Check sheet for the modelled part. Datum: model origin and axes. Units: mm. A direction names the side the tool comes from. Round coordinates to 2 decimals unless told otherwise and drop trailing zeros. Order: outer loops, then holes, each group sorted by start corner. A loop starts at its lowest first (then second) coordinate and runs counter-clockwise, first axis right, second up. Notation, with made-up numbers: (-15, -25.5) -> (32, -25.5) arc R16 cw to (32, -19.5) -> close; hole circle Ø8 at (24.25, 51). An arc over 180 degrees is marked (long way). Answer in a Markdown table with one row per item.
Autodesk Fusion 360 part; units mm, degrees
sketch "スケッチ1" plane through (0, 0, 0) normal (0, 0, 1) x (1, 0, 0)
  line L0 (0, 0) -> (72.6, 0)
  line L1 (72.6, 0) -> (72.6, -36.25)
  line L2 (72.6, -36.25) -> (0, -36.25)
  line L3 (0, -36.25) -> (0, 0)
  line L4 (36.3, 0) -> (36.3, -36.25)
  line L5 (0, -18.125) -> (72.6, -18.125)
  line L6 (72.6, -8.625) -> (72.6, -26.625)
  line L7 (58.3, -36.25) -> (14.3, -36.25)
  line L8 (0, -9.125) -> (0, -27.125)
  line L9 (0, -18.125) -> (9.5, -18.125)
  line L10 (0, -9.125) -> (6.4586, -9.125)
  line L11 (0, -27.125) -> (4.6488, -27.125)
  line L12 (6.4586, -9.125) -> (36.3, 0)
  line L13 (14.3, -36.25) -> (12.3, -36.25)
  line L14 (12.3, -36.25) -> (2.2204, -24.2289)
  line L15 (36.3, -18.125) -> (36.3, -32.425)
  line L16 (36.3, -18.125) -> (36.3, -3.825)
  line L17 (66.1414, -9.125) -> (36.3, 0)
  line L18 (60.3, -36.25) -> (70.3796, -24.2289)
  line L19 (58.3, -36.25) -> (60.3, -36.25)
  line L20 (6.4586, -27.125) -> (66.1414, -27.125)
  line L21 (6.4586, -9.125) -> (66.1414, -9.125)
  arc A0 (6.9878, -8.9632) -> (6.4586, -27.125) centre (9.5, -18.125) ccw
  arc A1 (66.1414, -27.125) -> (65.6122, -8.9632) centre (63.1, -18.125) ccw
  circle A2 centre (14.3, -32.425) radius 1.75
  circle A3 centre (36.3, -3.825) radius 1.75
  circle A4 centre (58.3, -32.425) radius 1.75
  circle A5 centre (32.3, -32.425) radius 1
  circle A6 centre (40.3, -32.425) radius 1
  point P0 (36.3, -18.125)
  point P1 (36.3, -3.825)
  point P2 (14.3, -32.425)
  point P3 (58.3, -32.425)
  point P4 (40.3, -32.425)
  point P5 (40.3, -32.425)
  point P6 (32.3, -32.425)
  dimension "d5" = 72.6
  dimension "d6" = 36.25
  dimension "d10" = 44
  dimension "d11" = 9
  dimension "d12" = 18
  dimension "d13" = 9.5
  dimension "d14" = 2
  dimension "d15" = 14.3
  dimension "d16" = 22
  dimension "d17" = 14.3
  dimension "d18" = 3.5
  dimension "d19" = 3.5
  dimension "d20" = 3.5
  dimension "d21" = 4
  dimension "d24" = 2
  dimension "d25" = 2
extrude "押し出し2" add sketch "スケッチ1" along normal blind 17 contours L4 L5 L9 L16 L21 A0 | L4 L5 L9 L15 L20 A0 | L4 L5 L16 L21 A1 | L4 L5 L15 L20 A1
sketch "スケッチ3" plane through (0, 0, 0) normal (0, 0, -1) x (1, 0, 0)
  arc A0 (6.4586, 27.125) -> (6.4586, 9.125) centre (9.5, 18.125) ccw
  line L0 (6.4586, 9.125) -> (66.1414, 9.125)
  arc A1 (66.1414, 9.125) -> (66.1414, 27.125) centre (63.1, 18.125) ccw
  line L1 (66.1414, 27.125) -> (6.4586, 27.125)
  line L2 (72.6, 18.125) -> (0, 18.125)
  line L3 (72.6, 18.125) -> (36.3, 18.125)
  line L4 (36.3, 18.125) -> (31.15, 18.125)
  line L5 (31.15, 18.125) -> (20.85, 18.125)
  line L6 (20.85, 18.125) -> (10.55, 18.125)
  line L7 (36.3, 18.125) -> (36.3, 27.125)
  point P0 (36.3, 18.125)
  point P1 (31.15, 18.125)
  point P2 (20.85, 18.125)
  point P3 (10.55, 18.125)
  point P4 (41.45, 18.125)
  point P5 (51.75, 18.125)
  point P6 (62.05, 18.125)
  dimension "d32" = 5.15
  dimension "d33" = 10.3
  dimension "d34" = 10.3
hole "穴1" at (62.05, -18.125, 0) at (51.75, -18.125, 0) at (41.45, -18.125, 0) at (31.15, -18.125, 0) at (20.85, -18.125, 0) at (10.55, -18.125, 0) direction (0, 0, 1) diameter 5 depth 23 tip angle 180
sketch "スケッチ4" plane through (0, 0, 17) normal (0, 0, 1) x (-1, 0, 0)
  circle A0 centre (-20.85, 18.125) radius 2.5
  circle A1 centre (-41.45, 18.125) radius 2.5
  circle A2 centre (-62.05, 18.125) radius 2.5
  circle A3 centre (-51.75, 18.125) radius 2.5
  circle A4 centre (-31.15, 18.125) radius 2.5
  circle A5 centre (-10.55, 18.125) radius 2.5
  arc A6 (-6.4586, 9.125) -> (-6.4586, 27.125) centre (-9.5, 18.125) ccw
  line L0 (-6.4586, 27.125) -> (-66.1414, 27.125)
  arc A7 (-66.1414, 27.125) -> (-66.1414, 9.125) centre (-63.1, 18.125) ccw
  line L1 (-66.1414, 9.125) -> (-6.4586, 9.125)
  line L2 (0, 18.125) -> (-4, 18.125)
  line L3 (-36.3, 13.125) -> (-5.4223, 13.125)
  line L4 (-4, 18.125) -> (-13.5, 18.125)
  line L5 (-36.3, 23.125) -> (-5.4223, 23.125)
  line L6 (-36.3, 23.125) -> (-36.3, 27.125)
  arc A8 (-5.4223, 13.125) -> (-5.4223, 23.125) centre (-13.5, 18.125) ccw
  line L7 (-36.3, 13.125) -> (-67.1777, 13.125)
  arc A9 (-67.1777, 23.125) -> (-67.1777, 13.125) centre (-59.1, 18.125) ccw
  line L8 (-36.3, 23.125) -> (-67.1777, 23.125)
  line L9 (-36.3, 23.125) -> (-36.3, 13.125)
  line L10 (-31.15, 18.125) -> (-41.45, 18.125)
  point P0 (-68.6, 18.125)
  dimension "d39" = 9.5
  dimension "d40" = 4
  dimension "d45" = 4
  dimension "d46" = 5
  dimension "d47" = 9.5
  dimension "d48" = 10.3
extrude "押し出し3" cut sketch "スケッチ4" against normal blind 15 contours A6 L0 L2 L5 L6 A8 | A6 L0 A7 L1 L2 L3 L6 A8 L7 A9 L8
fillet "フィレット2" radius 5 4 edges at (5.4223, -23.125, 9.5) (5.4223, -13.125, 9.5) (67.1777, -13.125, 9.5) (67.1777, -23.125, 9.5)
Item 1: Depth check by flat-ended pin: P1, Ø1, axis at y = -16, z = 6.5, coming from the +X side; P2, Ø1, axis at y = -19.5, z = 8, coming from the +X side; P3, Ø7.5, axis at x = 35.5, z = 7, coming from the +Y side (3 decimals). Enter the tip coordinate at first touch or a pass-through.
Result sheet:
| item | result |
|---|---|
| P1 | stops at x = 68.33 |
| P2 | stops at x = 68.52 |
| P3 | stops at y = -13.125 |
Item 2: Cross-section at C-C (y = -14.75). Record the boundary of the cut face in (x, z).
Result sheet:
| item | result |
|---|---|
| outline | (0.62, 0) -> (71.98, 0) -> (71.98, 2) -> (67.29, 2) -> (67.29, 17) -> (5.31, 17) -> (5.31, 2) -> (0.62, 2) -> close |
Item 3: Cross-section at A-A (x = 20.85). Record the boundary of the cut face in (y, z) (3 decimals).
Result sheet:
| item | result |
|---|---|
| outline | (-27.125, 0) -> (-20.625, 0) -> (-20.625, 17) -> (-23.125, 17) -> (-23.125, 2) -> (-27.125, 2) -> close; (-15.625, 0) -> (-9.125, 0) -> (-9.125, 2) -> (-13.125, 2) -> (-13.125, 17) -> (-15.625, 17) -> close |
Item 4: Mould release check, pull along Y, two halves, no side actions. Record for faces 4 (the cylindrical face through (63.57, -20.11, 8.62)), 5 (the cylindrical face through (67.174, -21.622, 9.395)), 6 (the cylindrical face through (10.44, -20.623, 8.619)), 7 (the flat face through (36, -18, 0)): pulls with the +Y half, pulls with the -Y half, needs draft (parallel to the pull), parting line crosses it, or undercut.
Result sheet:
| item | result |
|---|---|
| face 4 | undercut |
| face 5 | pulls with the -Y half |
| face 6 | undercut |
| face 7 | needs draft |
Item 5: Set-up check for faces 1 (the cylindrical face through (5.504, -21.7, 9.395)), 2 (the cylindrical face through (5.426, -14.628, 9.395)), 3 (the flat face through (36, -13.125, 10)): record each of +Z, -Z, +X, -X, +Y, -Y from which the full face is reachable in a straight line by a thin tool's end or side.
Result sheet:
| item | result |
|---|---|
| face 1 | +Z, -X, -Y |
| face 2 | +Z, -X, +Y |
| face 3 | +Z, +X, -X, +Y |
Item 6: Cross-section at B-B (z = 12.25). Record the boundary of the cut face in (x, y) (3 decimals).
Result sheet:
| item | result |
|---|---|
| outline | (4, -18.127) arc R4.999 ccw to (8.999, -23.125) -> (63.601, -23.125) arc R4.999 ccw to (68.6, -18.127) arc R9.5 ccw to (68.6, -18.123) arc R4.999 ccw to (63.601, -13.125) -> (8.999, -13.125) arc R4.999 ccw to (4, -18.123) arc R9.5 ccw to start; hole circle Ø5 at (10.55, -18.125); hole circle Ø5 at (20.85, -18.125); hole circle Ø5 at (31.15, -18.125); hole circle Ø5 at (41.45, -18.125); hole circle Ø5 at (51.75, -18.125); hole circle Ø5 at (62.05, -18.125) |
Item 7: Cross-section at D-D (x = 30.5). Record the boundary of the cut face in (y, z) (3 decimals), and give its area (3 significant figures).
Result sheet:
| item | result |
|---|---|
| outline | (-27.125, 0) -> (-20.539, 0) -> (-20.539, 17) -> (-23.125, 17) -> (-23.125, 2) -> (-27.125, 2) -> close; (-15.711, 0) -> (-9.125, 0) -> (-9.125, 2) -> (-13.125, 2) -> (-13.125, 17) -> (-15.711, 17) -> close |
| area | 104 mm^2 |
Item 8: Scan lines: line 1 (Y direction, x = 20.85, z = 13.75) (3 decimals); line 2 (Y direction, x = 59, z = 15) (3 decimals); line 3 (Y direction, x = 61, z = 16.25) (3 decimals). Record each from-to range of solid material in increasing order. Write a range as [from, to].
Result sheet:
| item | result |
|---|---|
| line 1 | y = [-23.125, -20.625], [-15.625, -13.125] |
| line 2 | y = [-23.125, -13.125] |
| line 3 | y = [-23.125, -20.394], [-15.856, -13.125] |
